Build history of the part. All positions in model axes, mm. A direction names the side the tool comes from. Round coordinates to 2 decimals unless told otherwise and drop trailing zeros. Order: outer loops, then holes, each group sorted by start corner. A loop starts at its lowest first (then second) coordinate and runs counter-clockwise, first axis right, second up. Notation, with made-up numbers: (1.5, 63.5) - (49.5, 63.5) arc R12 ccw to (49.5, 69.5) - close; hole circle Ø5 at (70, 49.25). An arc over 180 degrees is marked (long way). Write each question's results on one line, items separated by ' | '. Start each with the question number.
```python
from build123d import *

# Parameters (mm, degrees)
F2_R     = 9
F3_DEPTH = 25
F5_T     = 3.5
F6_D     = 6


# Not quite as in the source:
# - a shell that OpenCascade refuses in one call is made with other operations: the cavity is built on its own and cut out


with BuildPart() as f1:
    # F0 (on Right) → F1 (revolve)
    with BuildSketch(Plane.YZ):
        Polygon((0, 0), (25, 0), (25, 14), (20, 14), (15, 15), (10, 15), (10, 17), (0, 17), align=None)
    revolve(axis=Axis((0, 12.5, 0), (0, 1, 0)))

    # F2 (on Right) → F3 (cut, symmetric)
    with BuildSketch(Plane.YZ):
        with Locations((-0.5, 0)):
            Circle(F2_R)
    extrude(amount=F3_DEPTH, both=True, mode=Mode.SUBTRACT)

    # F5: shell of thickness 3.5, made by hand


with BuildPart() as f5_core1:
    # F5_t2: copy of F1
    add(f1.part)

    # the walls: a layer under each face that stays
    f5_faces = [f5_core1.faces().sort_by_distance(p)[0] for p in [
        (0, 22.5, -14),
        (0, 17.5, -14.5),
        (0, 12.5, -15),
        (-11.3333333333, 10, 11.3333333333),
        (0, 5, -17),
        (0, 0, -12.9930501889),
        (0, 8.5, 0),
        (0, 0, 12.9930501889),
    ]]
    thicken(f5_faces, amount=-F5_T, mode=Mode.SUBTRACT)

    # F5_s3 → F5_t4 (revolve, cut)
    with BuildSketch(Plane.YZ):
        Polygon((20.0068640647, 14.0693203236), (20, 10.5), (19.6534317024, 10.5), (19.313593527, 10.5679676351), align=None)
    revolve(axis=Axis((0, 20, 0), (0, 1, 0)), mode=Mode.SUBTRACT)

    # F5_s5 → F5_t6 (revolve, cut)
    with BuildSketch(Plane.YZ):
        Polygon((10.035, 15.035), (10, 11.5), (6.5, 11.5), (6.5, 15), align=None)
    revolve(axis=Axis((0, 10, 0), (0, 1, 0)), mode=Mode.SUBTRACT)


with BuildPart() as f1_1:
    add(f1.part)

    # what is left inside the walls is the cavity
    f5_cavity = [f5_core1.part.solids().sort_by_distance(p)[0] for p in [
        (-3.834029, 12.035, 0),
    ]]
    add(f5_cavity, mode=Mode.SUBTRACT)

    # F6 (through all)
    with Locations(Plane(origin=(0, 25, 0), x_dir=(-1, 0, 0), z_dir=(0, 1, 0))):
        with Locations((0, 0)):
            Hole(F6_D / 2)


solid = f1_1.part
```
1. Flat gauge pins, fed straight in: pin 1 Ø8 at (y, z) = (5, -13.5) entering from -X; pin 2 Ø1.5 at (x, y) = (2.5, 15) entering from -Z; pin 3 Ø4 at (x, y) = (13.5, 14) entering from -Z; pin 4 Ø5 at (y, z) = (3.5, -4) entering from -X. Where does each tip first touch, or does it go through?
2. Mould opens along X. For faces 4 (the face through (14.334, 4.93, 9.139)), 5 (the face through (0, 3.5, 12)), 6 (the face through (-14, 10, -6)) say: pulls with the +X half, pulls with the -X half, needs draft (parallel to the pull), parting line crosses it, or undercut.
3. 3-axis set-ups, long thin cutter, end or side, ignore diameter. For faces 1 (the face through (0.161, 11.582, 3.204)), 2 (the face through (3.2, 22.3, 10)), 3 (the face through (0.24, 7.93, -3.15)): which of +Z, -Z, +X, -X, +Y, -Y reach the whole face in a straight line?
4. Wall check: line 1 (X direction, y = 21.8, z = 0); line 2 (Z direction, x = 7.5, y = 9.25); line 3 (Y direction, x = -0.5, z = -13). Give the ranges that are in metal, low to high. Write a range as from..to.
5. Cut at B-B (y = 15.5). List the corners of the cut face in (x, z).
6. Cut at A-A (y = 23.75). List the corners of the cut face in (x, z).
A:
1) pin 1: stops at x = -14.1 | pin 2: stops at z = -14.9 | pin 3: stops at z = -9.63 | pin 4: passes through
2) face 4: parting line crosses it | face 5: undercut | face 6: needs draft
3) face 1: none | face 2: +Y | face 3: +X, -X, -Y
4) line 1: x = -14..-10.5, 10.5..14 | line 2: z = -15.26..-8.72, -7.82..7.82, 8.72..15.26 | line 3: y = 0..3.5, 6.5..25
5) outline: circle Ø29.8 at (0, 0); hole circle Ø22.66 at (0, 0)
6) outline: circle Ø28 at (0, 0); hole circle Ø21 at (0, 0)
